Read the model definition and answer for the solid it produces. Units are mm, in the model's axes. A direction names the side the tool comes from. Coordinates: 2 decimals unless noted, no trailing zeros. Order: outer loops, then holes, each group sorted by start corner. A loop starts at its lowest first (then second) coordinate and runs counter-clockwise, first axis right, second up. Notation, with made-up numbers: (82, 62.25) -> (131, 62.25) arc R21 ccw to (131, 99.25) -> close; hole circle Ø10 at (-16.5, 24.25). An arc over 180 degrees is marked (long way). Answer as a JSON object with one key per item and string values. Group by question number.
1) Given pin 1 (2 mm diameter, centred on y = 104, z = 18.5, fed in from +X); pin 2 (2.5 mm diameter, centred on y = 6.34, z = -5.66, fed in from -X); pin 3 (0.6 mm diameter, centred on x = 16, y = 107, fed in from +Z); pin 4 (1.6 mm diameter, centred on x = -16, z = -3.5, fed in from +Y), each flat-ended and moving along its own axis, determine where each tip first touches the part or whether it passes through.
2) Consider L1, parallel to Z at x = 16.3, y = 83.5; L2, parallel to Z at x = -3, y = 31; L3, parallel to X at y = 89.5, z = -17. Determine where each line is inside the solid, lowest interval first.
3) Section C-C on y = 51 is taken. Determine the outline of the cut face in (x, z), and give its area (3 significant figures).
4) Section A-A on x = -6 is taken. Determine the outline of the cut face in (y, z), and give its area (3 significant figures).
5) A tool of negligible diameter and unlimited length cuts with its end or side. For faces 1 (the flat face through (15.25, 76, 0)), 2 (the cylindrical face through (16.3, 80.8, 11.5)), 3 (the cylindrical face through (14.287, 119.248, -19.064)), 4 (the flat face through (19.75, 24, 0)), 5 (the cylindrical face through (-20.736, 4.811, -15.487)), from which of +Z, -Z, +X, -X, +Y, -Y can it reach the whole face along a straight path? Write none if from no direction.
6) Determine the mould class of faces 6 (the flat face through (-0.1, 125, -18.5)), 7 (the flat face through (19.5, 42.5, 0.3)), 8 (the cylindrical face through (-14.248, 80.713, 19.036)) for opening direction X: released by +X, released by -X, zero draft, split by the parting line, or undercut.
7) Section D-D on z = 15 is taken. Count the separate pieces of the cut face and the enclosed holes in it, and give its area (3 significant figures).
8) Section B-B on y = 77.2 is taken. Determine the outline of the cut face in (x, z).
from build123d import *

# Parameters (mm, degrees)
SKETCH1_W               = 43.5
SKETCH1_H               = 40.1
SKETCH1_W_2             = 39.5
SKETCH1_H_2             = 36.1
BOSS_EXTRUDE1_DEPTH     = 40
SKETCH3_R               = 1
SKETCH3_R_2             = 4.25
CUT_EXTRUDE2_DEPTH      = 44.5
SKETCH4_W               = 39.5
SKETCH4_H               = 30
CUT_EXTRUDE3_DEPTH      = 41.1
FILLET1_R               = 16
SKETCH8_W               = 43.5
SKETCH8_H               = 40.1
SKETCH7_W               = 34.5
SKETCH7_H               = 40.1
SKETCH11_W              = 30.5
SKETCH11_H              = 36.1
SKETCH10_W              = 39.5
SKETCH10_H              = 36.1
SKETCH12_W              = 34.5
SKETCH12_H              = 40.1
SKETCH12_W_2            = 30.5
SKETCH12_H_2            = 36.1
BOSS_EXTRUDE2_DEPTH     = 80
SKETCH5_W               = 24.33649167
SKETCH5_H               = 45
CUT_EXTRUDE4_DEPTH      = 5.5000001
CUT_EXTRUDE4_DEPTH_BACK = 40.0000001
SKETCH6_W               = 30
SKETCH6_H               = 40
CUT_EXTRUDE5_DEPTH      = 41.1000001
FILLET2_R               = 2
FILLET3_R               = 2.5
SKETCH16_R              = 1.35
CUT_EXTRUDE6_DEPTH      = 40.0000001


with BuildPart() as part:
    # Sketch1 → Boss-Extrude1 (new body)
    with BuildSketch(Plane(origin=(0, 0, 0), x_dir=(1, 0, 0), z_dir=(0, 1, 0))):
        Rectangle(SKETCH1_W, SKETCH1_H)
        Rectangle(SKETCH1_W_2, SKETCH1_H_2, mode=Mode.SUBTRACT)
    extrude(amount=BOSS_EXTRUDE1_DEPTH)

    # Sketch3 → Cut-Extrude2 (cut, through all)
    with BuildSketch(Plane(origin=(21.75, 0, 0), x_dir=(0, 0, -1), z_dir=(1, 0, 0))):
        with Locations((0, 20)):
            Circle(SKETCH3_R)
        with Locations((5.656854249, 17.656854249)):
            Circle(SKETCH3_R)
        with Locations((8, 12)):
            Circle(SKETCH3_R)
        with Locations((5.656854249, 6.343145751)):
            Circle(SKETCH3_R)
        with Locations((0, 4)):
            Circle(SKETCH3_R)
        with Locations((-5.656854249, 6.343145751)):
            Circle(SKETCH3_R)
        with Locations((-8, 12)):
            Circle(SKETCH3_R)
        with Locations((-5.656854249, 17.656854249)):
            Circle(SKETCH3_R)
        with Locations((0, 12)):
            Circle(SKETCH3_R_2)
    extrude(amount=-CUT_EXTRUDE2_DEPTH, mode=Mode.SUBTRACT)

    # Sketch4 → Cut-Extrude3 (cut, through all)
    with BuildSketch(Plane.XY.offset(20.05)):
        with Locations((0, 15)):
            Rectangle(SKETCH4_W, SKETCH4_H)
    extrude(amount=-CUT_EXTRUDE3_DEPTH, mode=Mode.SUBTRACT)

    # Fillet1
    fillet1_edges = [part.edges().sort_by_distance(p)[0] for p in [
        (20.75, 0, 20.05),
        (-20.75, 0, -20.05),
        (-20.75, 0, 20.05),
        (20.75, 0, -20.05),
    ]]
    fillet(fillet1_edges, radius=FILLET1_R)

    # Sketch8 → Loft2 section 0
    with BuildSketch(Plane(origin=(0, 40, 0), x_dir=(1, 0, 0), z_dir=(0, 1, 0))):
        Rectangle(SKETCH8_W, SKETCH8_H)
    # Sketch7 → Loft2 section 1
    with BuildSketch(Plane(origin=(0, 45, 0), x_dir=(1, 0, 0), z_dir=(0, 1, 0))):
        Rectangle(SKETCH7_W, SKETCH7_H)
    loft()

    # Sketch11 → Cut-Loft1 section 0
    with BuildSketch(Plane(origin=(0, 45, 0), x_dir=(1, 0, 0), z_dir=(0, 1, 0))):
        Rectangle(SKETCH11_W, SKETCH11_H)
    # Sketch10 → Cut-Loft1 section 1
    with BuildSketch(Plane(origin=(0, 40, 0), x_dir=(1, 0, 0), z_dir=(0, 1, 0))):
        Rectangle(SKETCH10_W, SKETCH10_H)
    loft(mode=Mode.SUBTRACT)

    # Sketch12 → Boss-Extrude2 (add)
    with BuildSketch(Plane(origin=(0, 45, 0), x_dir=(1, 0, 0), z_dir=(0, 1, 0))):
        Rectangle(SKETCH12_W, SKETCH12_H)
        Rectangle(SKETCH12_W_2, SKETCH12_H_2, mode=Mode.SUBTRACT)
    extrude(amount=BOSS_EXTRUDE2_DEPTH)

    # Sketch5 → Cut-Extrude4 (cut, two sides)
    with BuildSketch(Plane.ZY.offset(17.25)) as cut_extrude4_sk:
        with Locations((0, 102.5)):
            Rectangle(SKETCH5_W, SKETCH5_H)
    extrude(amount=CUT_EXTRUDE4_DEPTH, mode=Mode.SUBTRACT)
    extrude(cut_extrude4_sk.sketch, amount=-CUT_EXTRUDE4_DEPTH_BACK, mode=Mode.SUBTRACT)

    # Sketch6 → Cut-Extrude5 (cut, through all)
    with BuildSketch(Plane.XY.offset(20.05)):
        with Locations((0, 100)):
            Rectangle(SKETCH6_W, SKETCH6_H)
    extrude(amount=-CUT_EXTRUDE5_DEPTH, mode=Mode.SUBTRACT)

    # Fillet2
    fillet2_edges = [part.edges().sort_by_distance(p)[0] for p in [
        (-19.75, 30, 19.05),
        (19.75, 30, 19.05),
        (19.75, 30, -19.05),
        (-19.75, 30, -19.05),
        (-21.75, 40, 0),
        (17.25, 45, 0),
        (-17.25, 45, 0),
        (19.5, 42.5, 20.05),
        (-19.5, 42.5, 20.05),
        (19.5, 42.5, -20.05),
        (-19.5, 42.5, -20.05),
        (17.25, 85, -20.05),
        (-17.25, 85, -20.05),
        (-17.25, 85, 20.05),
        (17.25, 85, 20.05),
        (21.75, 40, 0),
    ]]
    fillet(fillet2_edges, radius=FILLET2_R)

    # Fillet3
    fillet3_edges = [part.edges().sort_by_distance(p)[0] for p in [
        (-19.75, 40, 0),
        (19.75, 40, 0),
        (15.25, 45, 0),
        (-15.25, 45, 0),
        (16.25, 80, -12.168245835),
        (16.25, 80, 12.168245835),
        (-15, 120, -19.05),
        (-15, 80, -19.05),
        (-16.25, 80, 12.168245835),
        (-16.25, 80, -12.168245835),
        (15, 80, -19.05),
        (15, 120, -19.05),
        (15, 120, 19.05),
        (-15, 120, 19.05),
        (-15, 80, 19.05),
        (15, 80, 19.05),
    ]]
    fillet(fillet3_edges, radius=FILLET3_R)

    # Sketch16 → Cut-Extrude6 (cut, through all)
    with BuildSketch(Plane.ZY.offset(17.25)):
        with Locations((-15.031754165, 117.5)):
            Circle(SKETCH16_R)
        with Locations((-15.031754165, 100.5)):
            Circle(SKETCH16_R)
        with Locations((-15.031754165, 83.5)):
            Circle(SKETCH16_R)
        with Locations((-8.531754165, 77.2)):
            Circle(SKETCH16_R)
        with Locations((8.468245835, 77.2)):
            Circle(SKETCH16_R)
        with Locations((14.968245835, 83.5)):
            Circle(SKETCH16_R)
        with Locations((14.968245835, 100.5)):
            Circle(SKETCH16_R)
        with Locations((14.968245835, 117.5)):
            Circle(SKETCH16_R)
    extrude(amount=-CUT_EXTRUDE6_DEPTH, mode=Mode.SUBTRACT)


solid = part.part
Worked answers:
{
 "1": {"pin 1": "stops at x = 17.25", "pin 2": "stops at x = -21.75", "pin 3": "stops at z = 20", "pin 4": "stops at y = 80"},
 "2": {"L1": "z = -19.75 to -16.38, -13.68 to -12.17, 12.17 to 13.62, 16.32 to 19.75", "L2": "z = -20.05 to -18.05, 18.05 to 20.05", "L3": "x = -17.25 to -15.25, 15.25 to 17.25"},
 "3": {"outline": "(-17.25, -18.05) arc R2 ccw to (-15.25, -20.05) -> (15.25, -20.05) arc R2 ccw to (17.25, -18.05) -> (17.25, 18.05) arc R2 ccw to (15.25, 20.05) -> (-15.25, 20.05) arc R2 ccw to (-17.25, 18.05) -> close; hole (-15.25, -18.05) -> (15.25, -18.05) -> (15.25, 18.05) -> (-15.25, 18.05) -> close", "area": "279 mm²"},
 "4": {"outline": "(30, -20.05) -> (80, -20.05) -> (80, -18.05) -> (30, -18.05) -> close; (30, 18.05) -> (80, 18.05) -> (80, 20.05) -> (30, 20.05) -> close; (120, -20.05) -> (125, -20.05) -> (125, -18.05) -> (120, -18.05) -> close; (120, 18.05) -> (125, 18.05) -> (125, 20.05) -> (120, 20.05) -> close", "area": "220 mm²"},
 "5": {"face 1": "+Y, -Y", "face 2": "+X, -X, +Y", "face 3": "+Z, -Z", "face 4": "-Y", "face 5": "-Z, +X, -X, -Y"},
 "6": {"face 6": "zero draft", "face 7": "released by +X", "face 8": "undercut"},
 "7": {"separate pieces": "8", "enclosed holes": "0", "area": "450 mm²"},
 "8": {"outline": "(-17.25, -18.05) arc R2 ccw to (-15.25, -20.05) -> (15.25, -20.05) arc R2 ccw to (17.25, -18.05) -> (17.25, -9.88) -> (15.25, -9.88) -> (15.25, -18.05) -> (-15.25, -18.05) -> (-15.25, -9.88) -> (-17.25, -9.88) -> close; (-17.25, -7.18) -> (-15.25, -7.18) -> (-15.25, 7.12) -> (-17.25, 7.12) -> close; (-17.25, 9.82) -> (-15.25, 9.82) -> (-15.25, 18.05) -> (15.25, 18.05) -> (15.25, 9.82) -> (17.25, 9.82) -> (17.25, 18.05) arc R2 ccw to (15.25, 20.05) -> (-15.25, 20.05) arc R2 ccw to (-17.25, 18.05) -> close; (15.25, -7.18) -> (17.25, -7.18) -> (17.25, 7.12) -> (15.25, 7.12) -> close"}
}
